```python
from build123d import *

# Parameters (mm, degrees)
SKETCH_1_W           = 7.25
SKETCH_1_H           = 6
EXTRUDE_1_DEPTH      = 7
SKETCH_2_W           = 5.85
SKETCH_2_H           = 4.6
CUT_EXTRUDE_1_DEPTH  = 5
SKETCH_3_W           = 0.7
SKETCH_3_H           = 0.8068671
SKETCH_3_W_2         = 3.039789906
SKETCH_3_H_2         = 0.7
CUT_EXTRUDE_2_DEPTH  = 5
EXTRUDE_2_DEPTH      = 4
EXTRUDE_2_DEPTH_BACK = 3.5
SKETCH_4_R           = 0.4


with BuildPart() as part:
    # 草图1 → 凸台-拉伸1 (new body)
    with BuildSketch(Plane.XY):
        with Locations((3.625, 3)):
            Rectangle(SKETCH_1_W, SKETCH_1_H)
    extrude(amount=EXTRUDE_1_DEPTH)

    # 草图2 → 切除-拉伸1 (cut)
    with BuildSketch(Plane.XY):
        with Locations((3.625, 3)):
            Rectangle(SKETCH_2_W, SKETCH_2_H)
    extrude(amount=CUT_EXTRUDE_1_DEPTH, mode=Mode.SUBTRACT)

    # 草图3 → 切除-拉伸2 (cut)
    with BuildSketch(Plane(origin=(0, 0, 0), x_dir=(-1, 0, 0), z_dir=(0, 0, -1))):
        with Locations((-6.9, 4.89656645)):
            Rectangle(SKETCH_3_W, SKETCH_3_H)
        with Locations((-0.35, 4.89656645)):
            Rectangle(SKETCH_3_W, SKETCH_3_H)
        with Locations((-3.625, 5.65)):
            Rectangle(SKETCH_3_W_2, SKETCH_3_H_2)
    extrude(amount=-CUT_EXTRUDE_2_DEPTH, mode=Mode.SUBTRACT)

    # 草图4 → 凸台-拉伸2 (add, two sides: drawn at the far end of the back side and taken through both)
    with BuildSketch(Plane(origin=(0, 0, 5), x_dir=(-1, 0, 0), z_dir=(0, 0, -1)).offset(-EXTRUDE_2_DEPTH_BACK)):
        with Locations((-4.875, 4)):
            Circle(SKETCH_4_R)
        with Locations((-2.375, 4)):
            Circle(SKETCH_4_R)
    extrude(amount=EXTRUDE_2_DEPTH + EXTRUDE_2_DEPTH_BACK)


solid = part.part
```
Model file for the job. Use its own axes, mm. A direction names the side the tool comes from. Coordinates: 2 decimals unless noted, no trailing zeros. Write each loop counter-clockwise with the first axis right and the second up, starting at its lowest first coordinate (ties: lowest second). Pieces come first, ordered by that corner, then holes. Notation, with made-up numbers: (57.5, 70) - (106.5, 70) arc R26 cw to (106.5, 94) - close; hole circle Ø9 at (38, 44). An arc over 180 degrees is marked (long way). Use a Markdown table: item, result. Add a question column.
Item 1: Band-saw the part on C-C, the plane z = 7.25. Write the cut outline in (x, y) (3 decimals).
Item 2: Band-saw the part on B-B, the plane y = 4. Write the cut outline in (x, z) (3 decimals).
Item 3: Drill centre lines: line 1 along X through (y, z) = (4.25, 4); line 2 along X through (y, z) = (4.1, 2.5); line 3 along Y through (x, z) = (0.75, 1.5). Where is each one in solid material? Low to high.
Item 4: Two-plate mould, pull along X, no slides. Class faces 5 (the face through (7.25, 3, 3)), 6 (the face through (5.17, 4.27, 7.76)), 7 (the face through (0, 3, 3)), 8 (the face through (3.6, 0.4, 0)): pulls with the +X half, pulls with the -X half, needs draft (parallel to the pull), parting line crosses it, or undercut.
Item 5: Band-saw the part on A-A, the plane x = 1.25. Write the cut outline in (y, z).
Item 6: 3-axis set-ups, long thin cutter, end or side, ignore diameter. For faces 1 (the face through (6, 5.3, 2)), 2 (the face through (4, 0, 3)), 3 (the face through (2.4, 4.4, 3)), 4 (the face through (2.4, 4.4, 7.8)): which of +Z, -Z, +X, -X, +Y, -Y reach the whole face in a straight line?
Item 7: Band-saw the part on D-D, the plane y = 5.5. Write the cut outline in (x, z), and give its area (3 significant figures).
Item 8: Drop flat-ended pins along their axis: pin 1 (2.5 mm diameter, centred on x = 2.5, z = 2, fed in from +Y); pin 2 (0.6 mm diameter, centred on x = 5, y = 4, fed in from -Z). Give the stop position or say it passes through.
A:
| question | item | result |
|---|---|---|
| 1 | outline | circle Ø0.8 at (2.375, 4); circle Ø0.8 at (4.875, 4) |
| 2 | outline | (0, 0) - (0.7, 0) - (0.7, 5) - (1.975, 5) - (1.975, 1) - (2.775, 1) - (2.775, 5) - (4.475, 5) - (4.475, 1) - (5.275, 1) - (5.275, 5) - (6.55, 5) - (6.55, 0) - (7.25, 0) - (7.25, 7) - (5.275, 7) - (5.275, 8.5) - (4.475, 8.5) - (4.475, 7) - (2.775, 7) - (2.775, 8.5) - (1.975, 8.5) - (1.975, 7) - (0, 7) - close |
| 3 | line 1 | x = 0 to 0.7, 2.06 to 2.69, 4.56 to 5.19, 6.55 to 7.25 |
| 3 | line 2 | x = 0 to 0.7, 1.99 to 2.76, 4.49 to 5.26, 6.55 to 7.25 |
| 3 | line 3 | y = 0 to 0.7, 5.3 to 6 |
| 4 | face 5 | pulls with the +X half |
| 4 | face 6 | undercut |
| 4 | face 7 | pulls with the -X half |
| 4 | face 8 | needs draft |
| 5 | outline | (0, 0) - (0.7, 0) - (0.7, 5) - (5.3, 5) - (5.3, 0) - (6, 0) - (6, 7) - (0, 7) - close |
| 6 | face 1 | -Z, +X, -X |
| 6 | face 2 | +Z, -Z, +X, -X, -Y |
| 6 | face 3 | -Z |
| 6 | face 4 | +Z |
| 7 | outline | (0, 0) - (2.11, 0) - (2.11, 5) - (5.14, 5) - (5.14, 0) - (7.25, 0) - (7.25, 7) - (0, 7) - close |
| 7 | area | 35.6 mm² |
| 8 | pin 1 | stops at y = 6 |
| 8 | pin 2 | stops at z = 1 |
